Check sheet for the modelled part. Datum: model origin and axes. Units: mm. A direction names the side the tool comes from. Give positions to 0.01 mm unless a question says otherwise; leave off trailing zeros. Order: outer loops, then holes, each group sorted by start corner. A loop starts at its lowest first (then second) coordinate and runs counter-clockwise, first axis right, second up.
```python
from build123d import *

# Parameters (mm, degrees)
F0_W      = 25.4
F0_H      = 25.399996
F1_DEPTH  = 4.572
F2_R      = 2.5
F3_DEPTH  = 4.318
F4_R      = 2.5
F5_DEPTH  = 4.064
F6_R      = 2.5
F7_DEPTH  = 3.81
F8_R      = 2.5
F9_DEPTH  = 3.556
F10_R     = 2.5
F11_DEPTH = 3.302


with BuildPart() as f1:
    # F0 (on Top) → F1 (new body)
    with BuildSketch(Plane.XY):
        Rectangle(F0_W, F0_H)
    extrude(amount=F1_DEPTH)

    # F2 (on face) → F3 (cut)
    with BuildSketch(Plane.XY.offset(4.572)):
        with Locations((-6.35, 6.35)):
            Circle(F2_R)
    extrude(amount=-F3_DEPTH, mode=Mode.SUBTRACT)

    # F4 (on face) → F5 (cut)
    with BuildSketch(Plane.XY.offset(4.572)):
        with Locations((6.35, 6.349998)):
            Circle(F4_R)
    extrude(amount=-F5_DEPTH, mode=Mode.SUBTRACT)

    # F6 (on face) → F7 (cut)
    with BuildSketch(Plane.XY.offset(4.572)):
        with Locations((-6.35, -6.349998)):
            Circle(F6_R)
    extrude(amount=-F7_DEPTH, mode=Mode.SUBTRACT)

    # F8 (on face) → F9 (cut)
    with BuildSketch(Plane.XY.offset(4.572)):
        with Locations((6.35, -6.349998)):
            Circle(F8_R)
    extrude(amount=-F9_DEPTH, mode=Mode.SUBTRACT)

    # F10 (on face) → F11 (cut)
    with BuildSketch(Plane.XY.offset(4.572)):
        Circle(F10_R)
    extrude(amount=-F11_DEPTH, mode=Mode.SUBTRACT)


solid = f1.part
```
(1) Cross-section at B-B on y = 0. Enter the section's corners in (x, z).
Response values:
outline: (-12.7, 0) - (12.7, 0) - (12.7, 4.57) - (2.5, 4.57) - (2.5, 1.27) - (-2.5, 1.27) - (-2.5, 4.57) - (-12.7, 4.57) - close
(2) Set-up check for faces 5 (the face through (-12.7, 0, 2)), 6 (the face through (0, 0, 1.27)): record each of +Z, -Z, +X, -X, +Y, -Y from which the full face is reachable in a straight line by a thin tool's end or side.
Response values:
face 5: +Z, -Z, -X, +Y, -Y
face 6: +Z
(3) Gauge pin test, flat ends, axial feed: pin 1 Ø2.5 at (x, y) = (6.5, 7) entering from +Z; pin 2 Ø4.5 at (x, y) = (-6.35, 6.35) entering from +Z; pin 3 Ø2.5 at (x, y) = (0.5, -0.5) entering from +Z. Record the tip position at first contact, or that the pin passes through.
Response values:
pin 1: stops at z = 0.51
pin 2: stops at z = 0.25
pin 3: stops at z = 1.27
(4) Cross-section at C-C on x = 6.35. Enter the section's corners in (y, z), then the cut area to 3 significant figures.
Response values:
outline: (-12.7, 0) - (12.7, 0) - (12.7, 4.57) - (8.85, 4.57) - (8.85, 0.51) - (3.85, 0.51) - (3.85, 4.57) - (-3.85, 4.57) - (-3.85, 1.02) - (-8.85, 1.02) - (-8.85, 4.57) - (-12.7, 4.57) - close
area: 78.0 mm2
(5) Cross-section at A-A on z = 3. Enter the section's corners in (x, y).
Response values:
outline: (-12.7, -12.7) - (12.7, -12.7) - (12.7, 12.7) - (-12.7, 12.7) - close; hole circle Ø5 at (-6.35, -6.35); hole circle Ø5 at (-6.35, 6.35); hole circle Ø5 at (0, 0); hole circle Ø5 at (6.35, -6.35); hole circle Ø5 at (6.35, 6.35)
(6) Material ranges on L1, parallel to Y at x = -6.35, z = 3.3; L2, parallel to Y at x = -8, z = 2.5; L3, parallel to X at y = 5.25, z = 3.3 (3 decimals), recorded low to high.
Response values:
L1: y = -12.7 to -8.85, -3.85 to 3.85, 8.85 to 12.7
L2: y = -12.7 to -8.23, -4.47 to 4.47, 8.23 to 12.7
L3: x = -12.7 to -8.595, -4.105 to 4.105, 8.595 to 12.7
(7) Cross-section at D-D on x = -6.35. Enter the section's corners in (y, z).
Response values:
outline: (-12.7, 0) - (12.7, 0) - (12.7, 4.57) - (8.85, 4.57) - (8.85, 0.25) - (3.85, 0.25) - (3.85, 4.57) - (-3.85, 4.57) - (-3.85, 0.76) - (-8.85, 0.76) - (-8.85, 4.57) - (-12.7, 4.57) - close
(8) Release check for a two-part mould opening along Y. For faces 1 (the face through (0, -12.7, 2)), 2 (the face through (0, 12.7, 2)), 3 (the face through (12.7, 0, 2)), 4 (the face through (6, 6, 0.508)) record: released by +Y, released by -Y, zero draft, split by the parting line, or undercut.
Response values:
face 1: released by -Y
face 2: released by +Y
face 3: zero draft
face 4: undercut
